Verification items for the finished model (mm, model axes). A direction names the side the tool comes from. Coordinates: 2 decimals unless noted, no trailing zeros. Order: outer loops, then holes, each group sorted by start corner. A loop starts at its lowest first (then second) coordinate and runs counter-clockwise, first axis right, second up. Notation, with made-up numbers: M 52,4.5 L 101,4.5 A16 ccw 101,28.5 Z; hole C -23,24.25 d5. An arc over 180 degrees is marked long. Answer as a JSON object with one key per item and string values. Group by question number.
(1) Mould release check, pull along Y, two halves, no side actions. Record for faces 1 (the face through (-0.325, -6.536, 7.395)), 2 (the face through (35, 0, 1)), 3 (the face through (-8, -10.5, 1)): released by +Y, released by -Y, zero draft, split by the parting line, or undercut.
(2) Cross-section at D-D (x = 32). Enter the section's corners in (y, z), plus the area to 3 significant figures.
(3) Cross-section at B-B (z = 11.5). Enter the section's corners in (x, y).
(4) Cross-section at C-C (x = 0). Enter the section's corners in (y, z), plus the area to 3 significant figures.
(5) Cross-section at A-A (y = 1). Enter the section's corners in (x, z), plus the area to 3 significant figures.
(6) Material ranges on line 1 (Y direction, x = 32, z = 0.8); line 2 (X direction, y = -17, z = 0.6); line 3 (X direction, y = -11, z = 9.25), recorded low to high.
(7) Gauge pin test, flat ends, axial feed: pin 1 Ø1.5 at (x, y) = (-6.5, -8) entering from +Z; pin 2 Ø5 at (y, z) = (-12.5, 5.5) entering from -X; pin 3 Ø1.6 at (x, z) = (-6.5, 1) entering from +Y; pin 4 Ø3 at (x, y) = (8, -13) entering from -Z. Record the tip position at first contact, or that the pin passes through.
(8) Access from +Z, -Z, +X, -X, +Y, -Y to the whole of each face (thin tool, end or side, straight path). Record for faces 4 (the face through (23, -10.5, 1)), 5 (the face through (-16.5, -8.07, 7.4)), 6 (the face through (-8, -5.5, 1)).
from build123d import *

# Parameters (mm, degrees)
SKETCH_W          = 70
SKETCH_H          = 5
PAD_DEPTH         = 2
PAD001_DEPTH      = 2
SKETCH002_R       = 3.3
PAD002_DEPTH      = 13
PAD002_DEPTH_BACK = 2
SKETCH003_R       = 1.5
SKETCH003_R_2     = 1.85
POCKET_DEPTH      = 15.001


with BuildPart() as part:
    # Sketch → Pad (new body)
    with BuildSketch(Plane.XY):
        with Locations((0, -8)):
            Rectangle(SKETCH_W, SKETCH_H)
    extrude(amount=PAD_DEPTH)

    # Sketch001 → Pad001 (new body)
    with BuildSketch(Plane.XY.offset(2)):
        with BuildLine():
            Line((35, 16.999981), (35, -17.000015))
            ThreePointArc((29, -17.000012), (31.999999, -20), (35, -17.000015))
            Line((29, -17.000012), (29, 16.999983))
            ThreePointArc((35, 16.999981), (32.000001, 20), (29, 16.999983))
        make_face()
    pad001 = extrude(amount=-PAD001_DEPTH)

    # Mirrored: Pad001 across Sketch001 V_Axis
    add(pad001.mirror(Plane(origin=(0, 0, 2), x_dir=(0, 0, 1), z_dir=(1, 0, 0))))

    # Sketch002 → Pad002 (new body, two sides)
    with BuildSketch(Plane.XY.offset(2)) as pad002_sk:
        with Locations((0, -8)):
            Circle(SKETCH002_R)
        with Locations((-15, -8)):
            Circle(SKETCH002_R)
        with Locations((15, -8)):
            Circle(SKETCH002_R)
    extrude(amount=PAD002_DEPTH)
    extrude(pad002_sk.sketch, amount=-PAD002_DEPTH_BACK)

    # Sketch003 → Pocket (cut, through all)
    with BuildSketch(Plane(origin=(0, 0, 0), x_dir=(1, 0, 0), z_dir=(0, 0, -1))):
        with Locations((0, 8)):
            Circle(SKETCH003_R)
        with Locations((-15, 8)):
            Circle(SKETCH003_R)
        with Locations((15, 8)):
            Circle(SKETCH003_R)
        with Locations((-32, -17)):
            Circle(SKETCH003_R_2)
        with Locations((-32, 17)):
            Circle(SKETCH003_R_2)
        with Locations((32, 17)):
            Circle(SKETCH003_R_2)
        with Locations((32, -17)):
            Circle(SKETCH003_R_2)
    extrude(amount=-POCKET_DEPTH, mode=Mode.SUBTRACT)


solid = part.part
Taken from the geometry:
{
 "1": {"face 1": "undercut", "face 2": "zero draft", "face 3": "released by -Y"},
 "2": {"outline": "M -20,0 L -18.85,0 L -18.85,2 L -20,2 Z; M -15.15,0 L 15.15,0 L 15.15,2 L -15.15,2 Z; M 18.85,0 L 20,0 L 20,2 L 18.85,2 Z", "area": "65.2 mm²"},
 "3": {"outline": "C -15,-8 d6.6; C 0,-8 d6.6; C 15,-8 d6.6; hole C -15,-8 d3; hole C 0,-8 d3; hole C 15,-8 d3"},
 "4": {"outline": "M -11.3,0 L -9.5,0 L -9.5,15 L -11.3,15 Z; M -6.5,0 L -4.7,0 L -4.7,15 L -6.5,15 Z", "area": "54.0 mm²"},
 "5": {"outline": "M -35,0 L -29,0 L -29,2 L -35,2 Z; M 29,0 L 35,0 L 35,2 L 29,2 Z", "area": "24.0 mm²"},
 "6": {"line 1": "y = -20 to -18.85, -15.15 to 15.15, 18.85 to 20", "line 2": "x = -35 to -33.85, -30.15 to -29, 29 to 30.15, 33.85 to 35", "line 3": "x = -16.37 to -13.63, -1.37 to 1.37, 13.63 to 16.37"},
 "7": {"pin 1": "stops at z = 2", "pin 2": "stops at x = -17.62", "pin 3": "stops at y = -5.5", "pin 4": "passes through"},
 "8": {"face 4": "+Z, -Z, -Y", "face 5": "+Z, -Z", "face 6": "+Z, -Z, +Y"}
}
